```python
from build123d import *

# Parameters (mm, degrees)
SKETCH2_R           = 0.25
BOSS_EXTRUDE1_DEPTH = 2


with BuildPart() as part:
    # Sketch1 → Revolve1 (revolve)
    with BuildSketch(Plane.XY, mode=Mode.PRIVATE) as revolve1_sk:
        with BuildLine():
            Line((0, 0), (0, 9))
            Line((0, 9), (-1, 9))
            ThreePointArc((-1, 9), (-1.707106781, 8.707106781), (-2, 8))
            Line((-2, 8), (-2, 6))
            Line((-2, 6), (-2, 1))
            Line((-2, 1), (-2.5, 1))
            Line((-2.5, 1), (-2.5, 0))
            Line((-2.5, 0), (0, 0))
        make_face()
    revolve(revolve1_sk.sketch.rotate(Axis((0, 0, 0), (0, 1, 0)), 270), axis=Axis((0, 0, 0), (0, 1, 0)))

    # Sketch2 → Boss-Extrude1 (add)
    with BuildSketch(Plane.XZ):
        with Locations(Location((1.5, 0, 0), (0, 0, 90))):
            Circle(SKETCH2_R)
        with Locations(Location((-1.5, 0, 0), (0, 0, 90))):
            Circle(SKETCH2_R)
    extrude(amount=BOSS_EXTRUDE1_DEPTH)


solid = part.part
```
Can you work these out from the model? Positions are in its coordinate system, mm. A direction names the side the tool comes from. Round coordinates to 2 decimals unless told otherwise and drop trailing zeros. Loops run counter-clockwise (first coordinate to the right, second up) from the corner with the lowest first, then second, coordinate; pieces in that order, holes last.
Item 1: Which directions (+Z, -Z, +X, -X, +Y, -Y) give clear straight access to the entire face, cutting with the end or side of a thin tool? Please do faces 1 (the cylindrical face through (2, 4, 0)), 2 (the cylindrical face through (2.44, 0.49, 0.54)).
Item 2: Please list where these lines run through material, in increasing order: L1, parallel to Y at x = -1.35, z = -1.6; L2, parallel to Y at x = 0.7, z = -0.15; L3, parallel to X at y = 7, z = -0.05.
Item 3: Will these pins go through, and if not, where does the flat tip stop? pin 1 Ø1.5 at (y, z) = (3.5, 1.5) entering from +X; pin 2 Ø3 at (x, z) = (1.5, -1) entering from +Y; pin 3 Ø1.5 at (x, z) = (0.5, -2) entering from +Y; pin 4 Ø1.5 at (x, z) = (0, 1) entering from -Y.
Item 4: Suppose I cut it at A-A, the plane y = 2.25. Write out the boundary of the cut face in (x, z).
Item 5: Suppose I cut it at B-B, the plane x = 2.2. Write out the boundary of the cut face in (y, z), then the cut area to 3 significant figures.
Reported:
1. face 1: +Y
1. face 2: +Y, -Y
2. L1: y = 0 to 1
2. L2: y = 0 to 9
2. L3: x = -2 to 2
3. pin 1: stops at x = 1.85
3. pin 2: stops at y = 9
3. pin 3: stops at y = 8.95
3. pin 4: stops at y = 0
4. outline: circle Ø4 at (0, 0)
5. outline: (0, -1.19) - (1, -1.19) - (1, 1.19) - (0, 1.19) - close
5. area: 2.37 mm2
